Part print with two shaded views. Sizes in mm from the minimum x, y, z corner. Round coordinates to 2 decimals unless told otherwise and drop trailing zeros. Loops run counter-clockwise (first coordinate to the right, second up) from the corner with the lowest first, then second, coordinate; pieces in that order, holes last. Notation, with made-up numbers: (67, 44.25) -> (116, 44.25) arc R9 ccw to (116, 51.25) -> close; hole circle Ø2 at (0, -35.5). An arc over 180 degrees is marked (long way). Answer as a JSON object with one key per item and string values. Group by question number.
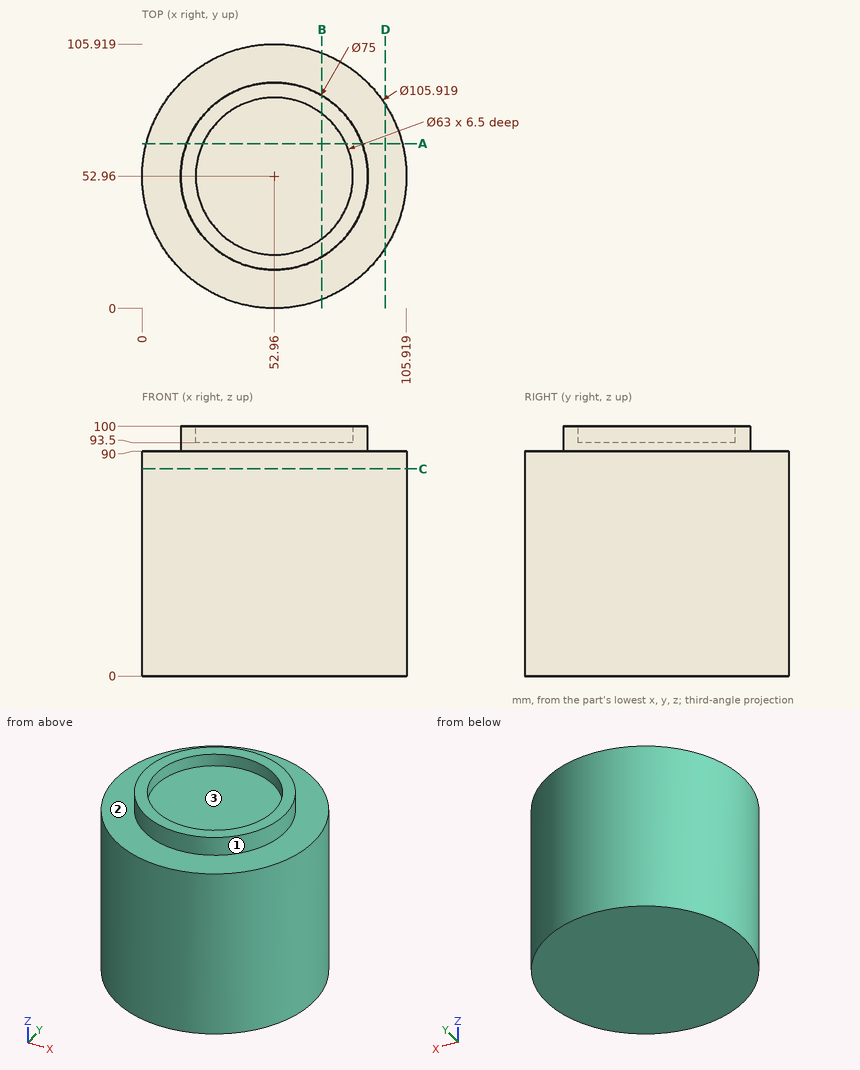
Item 1: Two-plate mould, pull along Y, no slides. Class the marked faces 1, 2 and 3: pulls with the +Y half, pulls with the -Y half, needs draft (parallel to the pull), parting line crosses it, or undercut.
Item 2: Band-saw the part on B-B, the plane x = 72. List the corners of the cut face in (y, z) (1 decimal).
Item 3: Band-saw the part on C-C, the plane z = 83. List the corners of the cut face in (x, y).
Item 4: Drill centre lines: line 1 (Z direction, x = 59.5, y = 90); line 2 (Z direction, x = 69, y = 35); line 3 (Y direction, x = 39, z = 94.5) (1 decimal). Where is each one in solid material? Low to high.
Item 5: Band-saw the part on D-D, the plane x = 97.5. List the corners of the cut face in (y, z).
Item 6: Drop flat-ended pins along their axis: pin 1 Ø6 at (x, z) = (34.5, 21.5) entering from +Y; pin 2 Ø3 at (x, z) = (47, 50) entering from -Y; pin 3 Ø2 at (x, y) = (80, 83.5) entering from -Z; pin 4 Ø10 at (y, z) = (40.5, 49) entering from -X. Give the stop position or say it passes through.
Item 7: Band-saw the part on A-A, the plane y = 66. List the corners of the cut face in (x, z) (1 decimal).
Entries:
{
 "1": {"face 1": "parting line crosses it", "face 2": "needs draft", "face 3": "undercut"},
 "2": {"outline": "(3.5, 0) -> (102.4, 0) -> (102.4, 90) -> (85.3, 90) -> (85.3, 100) -> (78.1, 100) -> (78.1, 93.5) -> (27.9, 93.5) -> (27.9, 100) -> (20.7, 100) -> (20.7, 90) -> (3.5, 90) -> close"},
 "3": {"outline": "circle Ø105.92 at (52.96, 52.96)"},
 "4": {"line 1": "0 to 90", "line 2": "0 to 93.5", "line 3": "18.2 to 24.7, 81.2 to 87.8"},
 "5": {"outline": "(24.31, 0) -> (81.61, 0) -> (81.61, 90) -> (24.31, 90) -> close"},
 "6": {"pin 1": "y = 103.61", "pin 2": "y = 0.19", "pin 3": "z = 0", "pin 4": "x = 0.53"},
 "7": {"outline": "(1.6, 0) -> (104.3, 0) -> (104.3, 90) -> (88.1, 90) -> (88.1, 100) -> (81.6, 100) -> (81.6, 93.5) -> (24.3, 93.5) -> (24.3, 100) -> (17.8, 100) -> (17.8, 90) -> (1.6, 90) -> close"}
}
